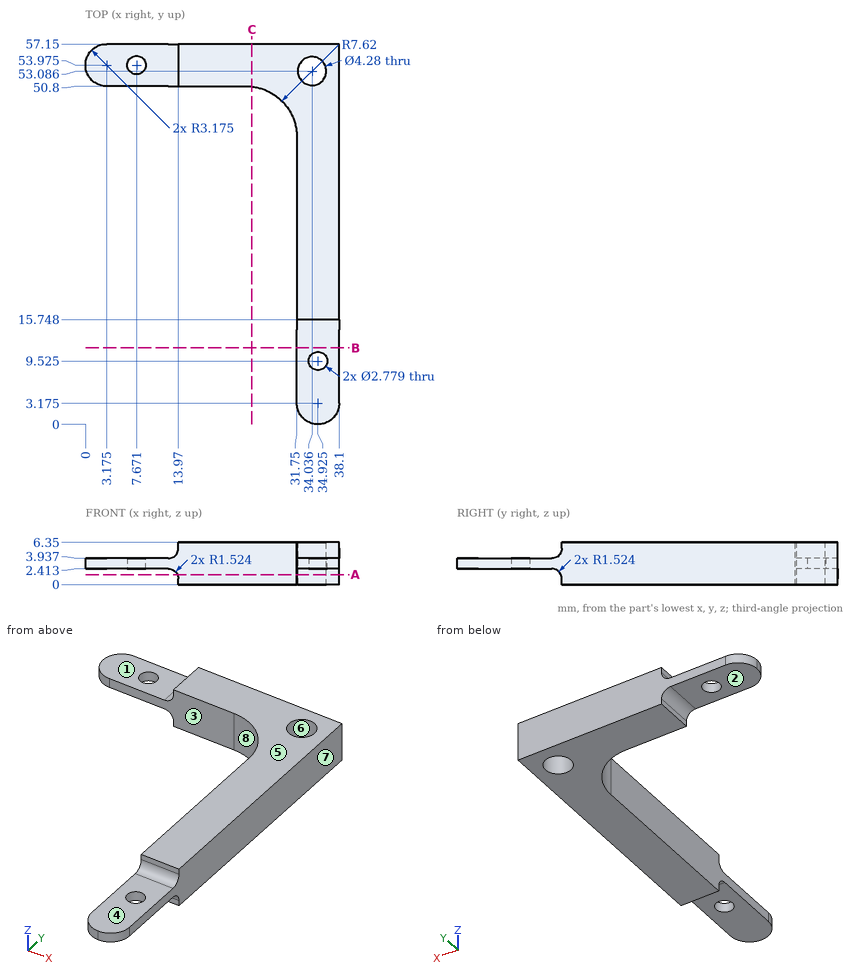
Could you check a few things on this drawing? It's one solid part, dimensions in mm from its lowest x, y, z. A direction names the side the tool comes from. Round coordinates to 2 decimals unless told otherwise and drop trailing zeros. Order: outer loops, then holes, each group sorted by start corner. A loop starts at its lowest first (then second) coordinate and runs counter-clockwise, first axis right, second up. Notation, with made-up numbers: M 54.5,83 L 83.5,83 A21 cw 83.5,109 Z; hole C 0,-15 d3. An arc over 180 degrees is marked long. Return JSON: item names as keys, results as strings. Group by question number.
1. Please list where these lines run through material, in increasing order: probe 1 along X at (y, z) = (38.5, 3.75); probe 2 along Y at (x, z) = (22, 2); probe 3 along X at (y, z) = (43.5, 4.25).
2. If we section it at C-C on x = 25: List the corners of the cut face in (y, z) for me.
3. If we mould it in two halves opening along X, with no side actions, what happens to the marked faces 5, 6, 7 and 8? For each: pulls with the +X half, pulls with the -X half, needs draft (parallel to the pull), parting line crosses it, or undercut.
4. If we section it at B-B on y = 11.5: List the corners of the cut face in (x, z) for me.
5. On a 3-axis mill with a long thin cutter (end or side, diameter ignored), from which of +Z, -Z, +X, -X, +Y, -Y can I reach the whole of each face in a straight line? I mean the marked faces 1, 2, 3 and 4. Say none if no direction works.
6. If we section it at A-A on z = 1.5: List the corners of the cut face in (x, y) for me.
7. I'm going to push flat-ended pins straight in: pin 1 Ø7 at (x, y) = (34.036, 53.086) entering from -Z; pin 2 Ø3 at (x, y) = (34.925, 9.525) entering from -Z; pin 3 Ø1 at (y, z) = (54, 0.5) entering from -X; pin 4 Ø3 at (x, z) = (16, 4.5) entering from -Y. Where does each tip first touch, or does it pass through?
Reply:
{
 "1": {"probe 1": "31.75 to 38.1", "probe 2": "50.8 to 57.15", "probe 3": "31.74 to 38.1"},
 "2": {"outline": "M 50.75,0 L 57.15,0 L 57.15,6.35 L 50.75,6.35 Z"},
 "3": {"face 5": "needs draft", "face 6": "undercut", "face 7": "pulls with the +X half", "face 8": "pulls with the -X half"},
 "4": {"outline": "M 31.75,2.41 L 38.1,2.41 L 38.1,3.94 L 31.75,3.94 Z"},
 "5": {"face 1": "+Z, -X, +Y, -Y", "face 2": "-Z, -X, +Y, -Y", "face 3": "+Z, -Z, -X, -Y", "face 4": "+Z, +X, -X, -Y"},
 "6": {"outline": "M 13.84,50.8 L 24.13,50.8 A7.62 cw 31.75,43.18 L 31.75,15.62 L 38.1,15.62 L 38.1,57.15 L 13.84,57.15 Z; hole C 34.04,53.09 d4.28"},
 "7": {"pin 1": "z = 0", "pin 2": "z = 2.41", "pin 3": "x = 13.97", "pin 4": "y = 50.8"}
}
